Source: CAD feature listing. Evaluate the final solid. Frame: model axes, mm. A direction names the side the tool comes from. Give positions to 0.01 mm unless a question says otherwise; leave off trailing zeros. Write each loop counter-clockwise with the first axis right and the second up, starting at its lowest first coordinate (ties: lowest second). Pieces come first, ordered by that corner, then holes.
```python
from build123d import *

# Parameters (mm, degrees)
SKETCH1_R                    = 20.5
SKETCH1_R_2                  = 7.5
BOSS_EXTRUDE1_DEPTH          = 3
SKETCH3_R                    = 1.4
CUT_EXTRUDE1_DEPTH           = 5
CHAMFER6_SIZE                = 0.3
CIRPATTERN2_COUNT            = 4
CHAMFER6_OF_CIRPATTERN2_SIZE = 0.3
SKETCH4_R                    = 20.5
SKETCH4_R_2                  = 1.4
SKETCH4_W                    = 1.5
SKETCH4_H                    = 1
BOSS_EXTRUDE2_DEPTH          = 60
SKETCH6_W                    = 1.5
SKETCH6_H                    = 1
BOSS_EXTRUDE4_DEPTH          = 15
FILLET1_R                    = 0.3
SKETCH7_R                    = 2.5
CUT_EXTRUDE2_DEPTH           = 1.5
SKETCH8_R                    = 0.85
CUT_EXTRUDE3_DEPTH           = 86.371248179
CHAMFER2_SIZE                = 0.2
CHAMFER4_SIZE                = 1
CHAMFER5_R                   = 0.2
SKETCH9_R                    = 1.4
CUT_EXTRUDE4_DEPTH           = 5


with BuildPart() as part:
    # Sketch1 → Boss-Extrude1 (new body)
    with BuildSketch(Plane(origin=(0, 0, 0), x_dir=(1, 0, 0), z_dir=(0, 1, 0))):
        with Locations(Location((0, 0, 0), (0, 0, 270))):
            Circle(SKETCH1_R)
        with Locations(Location((0, 0, 0), (0, 0, 270))):
            Circle(SKETCH1_R_2, mode=Mode.SUBTRACT)
    extrude(amount=BOSS_EXTRUDE1_DEPTH)

    # Sketch3 → Cut-Extrude1 (cut)
    with BuildSketch(Plane.XZ):
        with Locations(Location((0, 14.35, 0), (0, 0, 270))):
            Circle(SKETCH3_R)
    cut_extrude1 = extrude(amount=-CUT_EXTRUDE1_DEPTH, mode=Mode.SUBTRACT)

    # Chamfer6
    chamfer6_edges = [part.edges().sort_by_distance(p)[0] for p in [
        (0, 0, 15.75),
    ]]
    chamfer(chamfer6_edges, length=CHAMFER6_SIZE)

    # CirPattern2: Cut-Extrude1 ×4 about axis
    cirpattern2_axis = Axis((0, 0, 0), (0, 1, 0))
    for i in range(1, CIRPATTERN2_COUNT):
        add(cut_extrude1.rotate(cirpattern2_axis, i * 360 / CIRPATTERN2_COUNT), mode=Mode.SUBTRACT)

    # Chamfer6 of CirPattern2
    chamfer6_of_cirpattern2_edges = [part.edges().sort_by_distance(p)[0] for p in [
        (15.75, 0, 0),
        (0, 0, -15.75),
        (-15.75, 0, 0),
    ]]
    chamfer(chamfer6_of_cirpattern2_edges, length=CHAMFER6_OF_CIRPATTERN2_SIZE)

    # Sketch4 → Boss-Extrude2 (add)
    # profile 1 of 8: a face of its own
    with BuildSketch(Plane(origin=(0, 3, 0), x_dir=(1, 0, 0), z_dir=(0, 1, 0))):
        with Locations(Location((0, 0, 0), (0, 0, 270))):
            Circle(SKETCH4_R)
        with BuildLine():
            ThreePointArc((14.686303143, -11.25), (-3.697050438, -18.126825923), (-17.918984346, -4.6))
            ThreePointArc((-17.918984346, -4.6), (-2.318274099, 18.35417133), (18.5, 0))
            ThreePointArc((18.5, 0), (18.35417133, -2.318274099), (17.918984346, -4.6))
            ThreePointArc((17.918984346, -4.6), (16.751492877, -7.85095449), (15, -10.828203914))
            Line((15, -10.828203914), (15, -11.25))
            Line((15, -11.25), (14.686303143, -11.25))
        make_face(mode=Mode.SUBTRACT)
    # profile 2 of 8: a face of its own
    with BuildSketch(Plane(origin=(0, 3, 0), x_dir=(1, 0, 0), z_dir=(0, 1, 0))):
        with BuildLine():
            Line((-14.5, -7.5), (-14.5, -5.6))
            Line((-14.5, -5.6), (-14.5, -4.6))
            Line((-14.5, -4.6), (-17.918984346, -4.6))
            ThreePointArc((-17.918984346, -4.6), (-3.697050438, -18.126825923), (14.686303143, -11.25))
            Line((14.686303143, -11.25), (12, -11.25))
            Line((12, -11.25), (9, -11.25))
            Line((9, -11.25), (9, -10.25))
            Line((9, -10.25), (-13, -10.25))
            Line((-13, -10.25), (-13, -7.5))
            Line((-13, -7.5), (-14.5, -7.5))
        make_face()
        with Locations(Location((0, -14.35, 0), (0, 0, 270))):
            Circle(SKETCH4_R_2, mode=Mode.SUBTRACT)
    # profile 3 of 8: a face of its own
    with BuildSketch(Plane(origin=(0, 3, 0), x_dir=(1, 0, 0), z_dir=(0, 1, 0))):
        with BuildLine():
            Line((16.5, -4.6), (16.5, -5.6))
            Line((16.5, -5.6), (16.5, -7.5))
            Line((16.5, -7.5), (15, -7.5))
            Line((15, -7.5), (15, -10.25))
            Line((15, -10.25), (15, -10.828203914))
            ThreePointArc((15, -10.828203914), (16.751492877, -7.85095449), (17.918984346, -4.6))
            Line((17.918984346, -4.6), (16.5, -4.6))
        make_face()
    # profile 4 of 8: a face of its own
    with BuildSketch(Plane(origin=(0, 3, 0), x_dir=(1, 0, 0), z_dir=(0, 1, 0))):
        with BuildLine():
            Line((12, -11.25), (14.686303143, -11.25))
            ThreePointArc((14.686303143, -11.25), (14.844649762, -11.040216187), (15, -10.828203914))
            Line((15, -10.828203914), (15, -10.25))
            Line((15, -10.25), (12, -11.25))
        make_face()
    # profile 5 of 8: a face of its own
    with BuildSketch(Plane(origin=(0, 3, 0), x_dir=(1, 0, 0), z_dir=(0, 1, 0))):
        with Locations((15.75, -5.1)):
            Rectangle(SKETCH4_W, SKETCH4_H)
    # profile 6 of 8: a face of its own
    with BuildSketch(Plane(origin=(0, 3, 0), x_dir=(1, 0, 0), z_dir=(0, 1, 0))):
        with Locations((-13.75, -5.1)):
            Rectangle(SKETCH4_W, SKETCH4_H)
    # profile 7 of 8: a face of its own
    with BuildSketch(Plane(origin=(0, 3, 0), x_dir=(1, 0, 0), z_dir=(0, 1, 0))):
        with Locations(Location((0, -14.35, 0), (0, 0, 270))):
            Circle(SKETCH4_R_2)
    # profile 8 of 8: a face of its own
    with BuildSketch(Plane(origin=(0, 3, 0), x_dir=(1, 0, 0), z_dir=(0, 1, 0))):
        with BuildLine():
            ThreePointArc((15, -10.828203914), (14.844649762, -11.040216187), (14.686303143, -11.25))
            Line((14.686303143, -11.25), (15, -11.25))
            Line((15, -11.25), (15, -10.828203914))
        make_face()
    extrude(amount=BOSS_EXTRUDE2_DEPTH)

    # Sketch6 → Boss-Extrude4 (add)
    with BuildSketch(Plane(origin=(0, 63, 0), x_dir=(1, 0, 0), z_dir=(0, 1, 0))):
        with Locations((-13.75, -5.1)):
            Rectangle(SKETCH6_W, SKETCH6_H)
        with Locations((15.75, -5.1)):
            Rectangle(SKETCH6_W, SKETCH6_H)
        with BuildLine():
            Line((-14.5, -4.6), (-17.918984346, -4.6))
            ThreePointArc((-17.918984346, -4.6), (-3.697050438, -18.126825923), (14.686303143, -11.25))
            Line((14.686303143, -11.25), (12, -11.25))
            Line((12, -11.25), (9, -11.25))
            Line((9, -11.25), (9, -10.25))
            Line((9, -10.25), (-13, -10.25))
            Line((-13, -10.25), (-13, -7.5))
            Line((-13, -7.5), (-14.5, -7.5))
            Line((-14.5, -7.5), (-14.5, -5.6))
            Line((-14.5, -5.6), (-14.5, -4.6))
        make_face()
        with BuildLine():
            ThreePointArc((15, -10.828203914), (14.844649762, -11.040216187), (14.686303143, -11.25))
            Line((14.686303143, -11.25), (15, -11.25))
            Line((15, -11.25), (15, -10.828203914))
        make_face()
        with BuildLine():
            ThreePointArc((15, -10.828203914), (16.751492877, -7.85095449), (17.918984346, -4.6))
            Line((17.918984346, -4.6), (16.5, -4.6))
            Line((16.5, -4.6), (16.5, -5.6))
            Line((16.5, -5.6), (16.5, -7.5))
            Line((16.5, -7.5), (15, -7.5))
            Line((15, -7.5), (15, -10.25))
            Line((15, -10.25), (15, -10.828203914))
        make_face()
        with BuildLine():
            ThreePointArc((14.686303143, -11.25), (-3.697050438, -18.126825923), (-17.918984346, -4.6))
            Line((-17.918984346, -4.6), (-19.977237046, -4.6))
            ThreePointArc((-19.977237046, -4.6), (0, -20.5), (19.977237046, -4.6))
            Line((19.977237046, -4.6), (17.918984346, -4.6))
            ThreePointArc((17.918984346, -4.6), (16.751492877, -7.85095449), (15, -10.828203914))
            Line((15, -10.828203914), (15, -11.25))
            Line((15, -11.25), (14.686303143, -11.25))
        make_face()
        with BuildLine():
            Line((12, -11.25), (14.686303143, -11.25))
            ThreePointArc((14.686303143, -11.25), (14.844649762, -11.040216187), (15, -10.828203914))
            Line((15, -10.828203914), (15, -10.25))
            Line((15, -10.25), (12, -11.25))
        make_face()
    extrude(amount=BOSS_EXTRUDE4_DEPTH)

    # Fillet1
    fillet1_edges = [part.edges().sort_by_distance(p)[0] for p in [
        (15, 40.5, 4.6),
        (15, 40.5, 5.6),
        (16.5, 40.5, 5.6),
        (16.5, 40.5, 7.5),
        (15, 40.5, 7.5),
        (-13, 40.5, 10.25),
        (-13, 40.5, 7.5),
        (-14.5, 40.5, 7.5),
        (-14.5, 40.5, 5.6),
        (-13, 40.5, 5.6),
        (-13, 40.5, 4.6),
    ]]
    fillet(fillet1_edges, radius=FILLET1_R)

    # Sketch7 → Cut-Extrude2 (cut)
    with BuildSketch(Plane(origin=(0, 0, 4.6), x_dir=(-1, 0, 0), z_dir=(0, 0, -1))):
        with Locations((11.45, 71.2)):
            Circle(SKETCH7_R)
    cut_extrude2 = extrude(amount=-CUT_EXTRUDE2_DEPTH, mode=Mode.SUBTRACT)

    # Sketch8 → Cut-Extrude3 (cut, through all)
    with BuildSketch(Plane(origin=(0, 0, 7.5), x_dir=(-1, 0, 0), z_dir=(0, 0, -1))):
        with Locations((11.45, 71.2)):
            Circle(SKETCH8_R)
    cut_extrude3 = extrude(amount=-CUT_EXTRUDE3_DEPTH, mode=Mode.SUBTRACT)

    # Chamfer2
    chamfer2_edges = [part.edges().sort_by_distance(p)[0] for p in [
        (-10.6, 71.2, 10.25),
    ]]
    chamfer(chamfer2_edges, length=CHAMFER2_SIZE)

    # Mirror3: Cut-Extrude2, Cut-Extrude3 across plane
    add(cut_extrude2.mirror(Plane(origin=(1, 0, 0), x_dir=(0, 0, 1), z_dir=(1, 0, 0))), mode=Mode.SUBTRACT)
    add(cut_extrude3.mirror(Plane(origin=(1, 0, 0), x_dir=(0, 0, 1), z_dir=(1, 0, 0))), mode=Mode.SUBTRACT)

    # Chamfer4
    chamfer4_edges = [part.edges().sort_by_distance(p)[0] for p in [
        (9, 40.5, 10.25),
    ]]
    chamfer(chamfer4_edges, length=CHAMFER4_SIZE - 0.0001)  # a hair under: the kernel refuses the full size

    # Chamfer5
    chamfer5_edges = [part.edges().sort_by_distance(p)[0] for p in [
        (12.6, 71.199998189, 11.05),
    ]]
    fillet(chamfer5_edges, radius=CHAMFER5_R)

    # Sketch9 → Cut-Extrude4 (cut)
    with BuildSketch(Plane.XZ.offset(-3)):
        with Locations(Location((0, 14.35, 0), (0, 0, 270))):
            Circle(SKETCH9_R)
    extrude(amount=-CUT_EXTRUDE4_DEPTH, mode=Mode.SUBTRACT)


solid = part.part
```
1. Access query for faces 1 (the flat face through (0, 0, 9)), 2 (the cylindrical face through (0.06, 4.1, 15.75)), 3 (the flat face through (17, 48, 4.6)). Directions: +Z, -Z, +X, -X, +Y, -Y. A direction counts if a zero-diameter tool reaches every point of the face in a straight line with its end or side. Return the directions, or none.
2. Mould query, pull axis X, two halves, no side actions, for faces 4 (the cylindrical face through (-10.6, 71.2, 13.9)), 5 (the flat face through (-1, 63, -19)). Classes: +X half, -X half, draft (parallel to the pull), parting line (faces both ways), or undercut.
3. Line query: L1, parallel to X at y = 34, z = 0; L2, parallel to Y at x = 10, z = -15.5; L3, parallel to X at y = 25.5, z = -11. Output: solid intervals per line, ascending.
4. Cut plane B-B, the plane z = -14.35. Return the cut outline in (x, y), then the cut area to 3 significant figures.
5. Cut plane A-A, the plane x = 0. Return the cut outline in (y, z), then the cut area to 3 significant figures.
6. Contact query for flat-ended pins moving along their axis: P1, Ø0.6, axis at y = 24.5, z = 9, coming from the +X side; P2, Ø0.7, axis at y = 42, z = 6.5, coming from the -X side; P3, Ø1, axis at x = -11.45, y = 71.2, coming from the -Z side; P4, Ø1, axis at x = -14, y = 41, coming from the -Z side. Output: stop coordinate, or through.
7. Cut plane D-D, the plane z = 3. Return the cut outline in (x, y).
Response values:
1. face 1: +Z, -Z, +X, -X, -Y
1. face 2: -Y
1. face 3: +Y
2. face 4: undercut
2. face 5: draft
3. L1: x = -20.5 to -18.5, 18.5 to 20.5
3. L2: y = 0 to 3
3. L3: x = -17.3 to -14.87, 14.87 to 17.3
4. outline: (-14.64, 0) - (-1.7, 0) - (-1.4, 0.3) - (-1.4, 3) - (-11.68, 3) - (-11.68, 63) - (-14.64, 63) - close; (1.4, 0.3) - (1.7, 0) - (14.64, 0) - (14.64, 63) - (11.68, 63) - (11.68, 3) - (1.4, 3) - close
4. area: 435 mm2
5. outline: (0, -20.5) - (63, -20.5) - (63, -18.5) - (3, -18.5) - (3, -15.75) - (0.3, -15.75) - (0, -16.05) - close; (0, -12.65) - (0.3, -12.95) - (3, -12.95) - (3, -7.5) - (0, -7.5) - close; (0, 7.5) - (3, 7.5) - (3, 10.25) - (78, 10.25) - (78, 20.5) - (0, 20.5) - (0, 16.05) - (0.3, 15.75) - (8, 15.75) - (8, 12.95) - (0.3, 12.95) - (0, 12.65) - close
5. area: 936 mm2
6. P1: stops at x = 18.56
6. P2: stops at x = -19.56
6. P3: passes through
6. P4: stops at z = -15.43
7. outline: (-20.28, 0) - (-6.87, 0) - (-6.87, 3) - (-18.26, 3) - (-18.26, 63) - (-20.28, 63) - close; (6.87, 0) - (20.28, 0) - (20.28, 63) - (18.26, 63) - (18.26, 3) - (6.87, 3) - close
